from build123d import *

# Parameters (mm, degrees)
BOSS_EXTRUDE1_DEPTH = 50
SKETCH2_R           = 1.75
CUT_EXTRUDE1_DEPTH  = 72.941382389
CUT_EXTRUDE2_DEPTH  = 8.249997


with BuildPart() as part:
    # Sketch1 → Boss-Extrude1 (new body)
    with BuildSketch(Plane.XY):
        with BuildLine():
            Line((50, 10.224622738), (50, 5.224622738))
            ThreePointArc((50, 5.224622738), (45, 3.884876776), (41.339745962, 0.224622738))
            ThreePointArc((41.339745962, 0.224622738), (38.927083678, -2.096523604), (35.710580838, -3.025377262))
            Line((35.710580838, -3.025377262), (14.289419162, -3.025377262))
            ThreePointArc((14.289419162, -3.025377262), (11.039419162, -2.154542386), (8.660254038, 0.224622738))
            ThreePointArc((8.660254038, 0.224622738), (5, 3.884876776), (0, 5.224622738))
            Line((0, 5.224622738), (0, 10.224622738))
            Line((0, 10.224622738), (14.25, 10.224622738))
            Line((14.25, 10.224622738), (14.25, 3.724622738))
            ThreePointArc((14.25, 3.724622738), (14.762563133, 2.487185871), (16, 1.974622738))
            Line((16, 1.974622738), (34, 1.974622738))
            ThreePointArc((34, 1.974622738), (35.237436867, 2.487185871), (35.75, 3.724622738))
            Line((35.75, 3.724622738), (35.75, 10.224622738))
            Line((35.75, 10.224622738), (50, 10.224622738))
        make_face()
    extrude(amount=-BOSS_EXTRUDE1_DEPTH)

    # Sketch2 → Cut-Extrude1 (cut, through all)
    with BuildSketch(Plane.XZ.offset(3.025377262)):
        with Locations(Location((6.75, -43.25, 0), (0, 0, 270))):
            Circle(SKETCH2_R)
        with Locations(Location((43.25, -43.25, 0), (0, 0, 270))):
            Circle(SKETCH2_R)
        with Locations(Location((6.75, -6.75, 0), (0, 0, 270))):
            Circle(SKETCH2_R)
        with Locations(Location((43.25, -6.75, 0), (0, 0, 270))):
            Circle(SKETCH2_R)
    extrude(amount=-CUT_EXTRUDE1_DEPTH, mode=Mode.SUBTRACT)

    # Sketch3 → Cut-Extrude2 (cut)
    with BuildSketch(Plane.XZ.offset(3.025377262)):
        Polygon((9.75, -5.017949192), (6.75, -3.285898385), (3.75, -5.017949192), (3.75, -8.482050808), (6.75, -10.214101615), (9.75, -8.482050808), align=None)
        Polygon((6.770844829, -39.785961101), (3.760476728, -41.499928399), (3.739631899, -44.963967298), (6.729155171, -46.714038899), (9.739523272, -45.000071601), (9.760368101, -41.536032702), align=None)
        Polygon((40.239631899, -41.536032702), (43.229155171, -39.785961101), (46.239523272, -41.499928399), (46.260368101, -44.963967298), (43.270844829, -46.714038899), (40.260476728, -45.000071601), align=None)
        Polygon((40.25, -8.482050808), (40.25, -5.017949192), (43.25, -3.285898385), (46.25, -5.017949192), (46.25, -8.482050808), (43.25, -10.214101615), align=None)
    extrude(amount=-CUT_EXTRUDE2_DEPTH, mode=Mode.SUBTRACT)


solid = part.part
For this review, take the finished solid that the model builds, in its own axes (mm). A direction names the side the tool comes from. Give positions to 0.01 mm unless a question says otherwise; leave off trailing zeros. Order: outer loops, then holes, each group sorted by start corner. A loop starts at its lowest first (then second) coordinate and runs counter-clockwise, first axis right, second up. Notation, with made-up numbers: (76.5, -37.5) - (133.5, -37.5) arc R26 ccw to (133.5, -22.5) - close; hole circle Ø1 at (82, 25). An arc over 180 degrees is marked (long way). Answer as a JSON object with one key per item and string values. Group by question number.
Item 1: Wall thickness on line 1 along X through (y, z) = (6.7, -6.75); line 2 along X through (y, z) = (6.5, -21.5); line 3 along X through (y, z) = (8, -8): over which ranges is each line inside the solid? List them lowest first.
Item 2: Clearance check with flat-ended pins moving along their axes: pin 1 Ø2 at (y, z) = (3, -35) entering from +X; pin 2 Ø9 at (x, z) = (21, -22) entering from +Y; pin 3 Ø1.8 at (x, z) = (6.5, -42) entering from -Y. State where each tip first meets the part, or that it passes through.
Item 3: Take a section at A-A on y = 7.75. Give the boundary of the cut face in (x, z), and give its area (3 significant figures).
Item 4: Take a section at B-B on z = -43.25. Give the boundary of the cut face in (x, y).
Item 5: Take a section at D-D on x = 29.5. Give the boundary of the cut face in (y, z).
Item 6: Machinability: for faces 1 (the flat face through (25, 1, -50)), 2 (the cylindrical face through (14.75, 2.5, -24.65)), 3 (the flat face through (5.62, 4.47, -40.44)), which of the approach directions +Z, -Z, +X, -X, +Y, -Y give a long, thin tool a straight path to every point of the face, cutting with its end or side? Answer none if there is none.
Item 7: Draft analysis for pull direction Z (two halves, no side actions). For faces 4 (the flat face through (5.562, 4.478, -9.528)), 5 (the flat face through (8, 5.225, -45)), 6 (the flat face through (35.75, 7, -25)), 7 (the flat face through (25, 1, 0)), state which applies: pulls with the +Z half, pulls with the -Z half, needs draft (parallel to the pull), parting line crosses it, or undercut.
Item 8: Take a section at C-C on z = -17. Give the boundary of the cut face in (x, y).
Reported:
{
 "1": {"line 1": "0 to 5, 8.5 to 14.25, 35.75 to 41.5, 45 to 50", "line 2": "0 to 14.25, 35.75 to 50", "line 3": "0 to 5.53, 7.97 to 14.25, 35.75 to 42.03, 44.47 to 50"},
 "2": {"pin 1": "x = 45.2", "pin 2": "y = 1.97", "pin 3": "y = 5.22"},
 "3": {"outline": "(0, -50) - (14.25, -50) - (14.25, 0) - (0, 0) - close; (35.75, -50) - (50, -50) - (50, 0) - (35.75, 0) - close; hole circle Ø3.5 at (6.75, -43.25); hole circle Ø3.5 at (6.75, -6.75); hole circle Ø3.5 at (43.25, -43.25); hole circle Ø3.5 at (43.25, -6.75)", "area": "1,390 mm^2"},
 "4": {"outline": "(0, 5.22) arc R10 cw to (3.75, 4.49) - (3.75, 5.22) - (5, 5.22) - (5, 10.22) - (0, 10.22) - close; (8.5, 5.22) - (9.75, 5.22) - (9.75, -1.18) arc R6.5 ccw to (14.29, -3.03) - (35.71, -3.03) arc R6.97 ccw to (40.25, -1.11) - (40.25, 5.22) - (41.5, 5.22) - (41.5, 10.22) - (35.75, 10.22) - (35.75, 3.72) arc R1.75 cw to (34, 1.97) - (16, 1.97) arc R1.75 cw to (14.25, 3.72) - (14.25, 10.22) - (8.5, 10.22) - close; (45, 5.22) - (46.25, 5.22) - (46.25, 4.49) arc R10 cw to (50, 5.22) - (50, 10.22) - (45, 10.22) - close"},
 "5": {"outline": "(-3.03, -50) - (1.97, -50) - (1.97, 0) - (-3.03, 0) - close"},
 "6": {"face 1": "-Z, +X, -X, +Y, -Y", "face 2": "+Z, -Z, +Y", "face 3": "-Y"},
 "7": {"face 4": "undercut", "face 5": "undercut", "face 6": "needs draft", "face 7": "pulls with the +Z half"},
 "8": {"outline": "(0, 5.22) arc R10 cw to (8.66, 0.22) arc R6.5 ccw to (14.29, -3.03) - (35.71, -3.03) arc R6.97 ccw to (41.34, 0.22) arc R10 cw to (50, 5.22) - (50, 10.22) - (35.75, 10.22) - (35.75, 3.72) arc R1.75 cw to (34, 1.97) - (16, 1.97) arc R1.75 cw to (14.25, 3.72) - (14.25, 10.22) - (0, 10.22) - close"}
}
